Source: CAD feature listing. Evaluate the final solid. Frame: model axes, mm. Round coordinates to 2 decimals unless told otherwise and drop trailing zeros. Loops run counter-clockwise (first coordinate to the right, second up) from the corner with the lowest first, then second, coordinate; pieces in that order, holes last. Notation, with made-up numbers: (71, 29) -> (83, 29) arc R11 cw to (83, 35) -> close; hole circle Ø3 at (52, 29). An arc over 180 degrees is marked (long way). Write item = value, one per line.
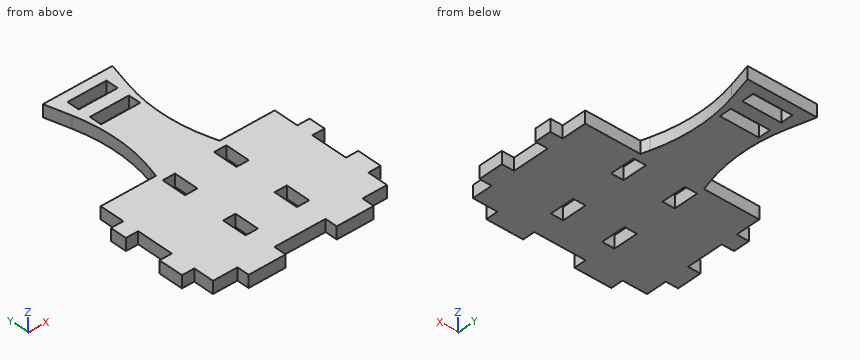
from build123d import *

# Parameters (mm, degrees)
SKETCH1_W           = 6
SKETCH1_H           = 12
SKETCH1_W_2         = 19.012644139
SKETCH1_H_2         = 6
BOSS_EXTRUDE1_DEPTH = 6


with BuildPart() as part:
    # Sketch1 → Boss-Extrude1 (new body)
    with BuildSketch(Plane.XY):
        with BuildLine():
            Line((-71.009489367, -30.923530446), (-71.009489367, -48.923530446))
            Line((-71.009489367, -48.923530446), (-77.009489367, -48.923530446))
            Line((-77.009489367, -48.923530446), (-77.009489367, -60.923530446))
            Line((-77.009489367, -60.923530446), (-71.009489367, -60.923530446))
            Line((-71.009489367, -60.923530446), (-71.009489367, -70.923530446))
            Line((-71.009489367, -70.923530446), (-59.069535867, -70.923530446))
            Line((-59.069535867, -70.923530446), (-59.069535867, -76.923530446))
            Line((-59.069535867, -76.923530446), (-41.069535867, -76.923530446))
            Line((-41.069535867, -76.923530446), (-41.069535867, -70.923530446))
            Line((-41.069535867, -70.923530446), (-16.155263667, -70.923530446))
            Line((-16.155263667, -70.923530446), (-16.155263667, -76.923530446))
            Line((-16.155263667, -76.923530446), (1.844736333, -76.923530446))
            Line((1.844736333, -76.923530446), (1.844736333, -70.923530446))
            Line((1.844736333, -70.923530446), (13.784689833, -70.923530446))
            Line((13.784689833, -70.923530446), (13.784689833, -60.923530446))
            Line((13.784689833, -60.923530446), (19.784689833, -60.923530446))
            Line((19.784689833, -60.923530446), (19.784689833, -48.923530446))
            Line((19.784689833, -48.923530446), (13.784689833, -48.923530446))
            Line((13.784689833, -48.923530446), (13.784689833, -30.923530446))
            Line((13.784689833, -30.923530446), (19.784689833, -30.923530446))
            Line((19.784689833, -30.923530446), (19.784689833, -22.923530446))
            Line((19.784689833, -22.923530446), (13.784689833, -22.923530446))
            Line((13.784689833, -22.923530446), (13.784689833, -10.85146976))
            Line((13.784689833, -10.85146976), (-13.112399767, -10.85146976))
            Line((-13.112399767, -10.85146976), (-14.257146074, -6.967198767))
            ThreePointArc((-14.257146074, -6.967198767), (-17.512012302, 14.497312555), (-14.875995677, 36.046577434))
            Line((-14.875995677, 36.046577434), (-11.701450566, 48.085223564))
            Line((-11.701450566, 48.085223564), (-45.510704829, 48.085223564))
            Line((-45.510704829, 48.085223564), (-42.338764303, 36.045890917))
            ThreePointArc((-42.338764303, 36.045890917), (-39.707407485, 14.496217042), (-42.966828756, -6.967441914))
            Line((-42.966828756, -6.967441914), (-44.112399767, -10.85146976))
            Line((-44.112399767, -10.85146976), (-71.009489367, -10.85146976))
            Line((-71.009489367, -10.85146976), (-71.009489367, -22.923530446))
            Line((-71.009489367, -22.923530446), (-77.009489367, -22.923530446))
            Line((-77.009489367, -22.923530446), (-77.009489367, -30.923530446))
            Line((-77.009489367, -30.923530446), (-71.009489367, -30.923530446))
        make_face()
        with Locations((-41.112399767, -52.830649895)):
            Rectangle(SKETCH1_W, SKETCH1_H, mode=Mode.SUBTRACT)
        with Locations((-41.112399767, -20.484459594)):
            Rectangle(SKETCH1_W, SKETCH1_H, mode=Mode.SUBTRACT)
        with Locations((-16.112399767, -20.484459594)):
            Rectangle(SKETCH1_W, SKETCH1_H, mode=Mode.SUBTRACT)
        with Locations((-16.112399767, -52.830649895)):
            Rectangle(SKETCH1_W, SKETCH1_H, mode=Mode.SUBTRACT)
        with Locations((-28.606077697, 40.085223564)):
            Rectangle(SKETCH1_W_2, SKETCH1_H_2, mode=Mode.SUBTRACT)
        with Locations((-28.606077697, 28.085223564)):
            Rectangle(SKETCH1_W_2, SKETCH1_H_2, mode=Mode.SUBTRACT)
    extrude(amount=BOSS_EXTRUDE1_DEPTH)


solid = part.part
1. Section query B-B (z = 2.55). Give the number of separate pieces and of enclosed holes in the cut face, then the cut area to 3 significant figures.
Evaluation:
separate_pieces = 1
enclosed_holes = 6
area = 6,560 mm²
2. Section query C-C (x = -66.5). Return the cut outline in (y, z), then the cut area to 3 significant figures.
Evaluation:
outline = (-70.92, 0) -> (-10.85, 0) -> (-10.85, 6) -> (-70.92, 6) -> close
area = 360 mm²
3. Section query A-A (x = -35.5). Return the cut outline in (y, z).
Evaluation:
outline = (-70.92, 0) -> (25.09, 0) -> (25.09, 6) -> (-70.92, 6) -> close; (31.09, 0) -> (37.09, 0) -> (37.09, 6) -> (31.09, 6) -> close; (43.09, 0) -> (48.09, 0) -> (48.09, 6) -> (43.09, 6) -> close
4. Contact query for flat-ended pins moving along their axis: pin 1 Ø8 at (x, y) = (-39.5, -38) entering from -Z; pin 2 Ø3 at (x, z) = (5, 3) entering from -Y; pin 3 Ø1.8 at (y, z) = (-65.5, 3) entering from -X; pin 4 Ø3 at (x, z) = (-6, 3) entering from +Y. Output: stop coordinate, or through.
Evaluation:
pin_1 = 0
pin_2 = -70.92
pin_3 = -71.01
pin_4 = -10.85
5. Line query: probe 1 along Y at (x, z) = (-19.5, 5.75); probe 2 along X at (y, z) = (-53, 3.9); probe 3 along X at (y, z) = (14, 3). Output: solid intervals per line, ascending. Write a range as from..to.
Evaluation:
probe_1 = -70.92..25.09, 31.09..37.09, 43.09..48.09
probe_2 = -77.01..-44.11, -38.11..-19.11, -13.11..19.78
probe_3 = -39.72..-17.5
6. Section query D-D (y = -33.5). Return the cut outline in (x, z), then the cut area to 3 significant figures.
Evaluation:
outline = (-71.01, 0) -> (13.78, 0) -> (13.78, 6) -> (-71.01, 6) -> close
area = 509 mm²
